```python
from build123d import *

# Parameters (mm, degrees)
F0_W     = 12.7
F0_H     = 44.45
F1_DEPTH = 12.7


with BuildPart() as f1:
    # F0 (on Top) → F1 (new body)
    with BuildSketch(Plane.XY):
        Rectangle(F0_W, F0_H)
        with BuildLine():
            Line((6.35, -22.225), (-6.35, -22.225))
            ThreePointArc((-6.35, -22.225), (-15.875, -31.75), (-25.4, -22.225))
            Line((-25.4, -22.225), (-38.1, -22.225))
            ThreePointArc((-38.1, -22.225), (-15.875, -44.45), (6.35, -22.225))
        make_face()
    extrude(amount=F1_DEPTH)


solid = f1.part
```
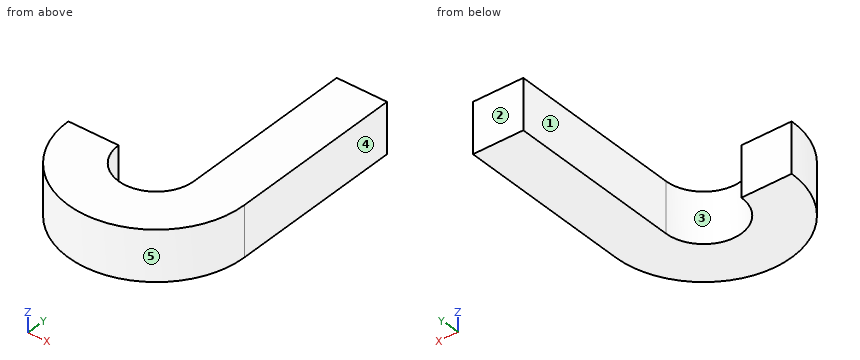
The model under review builds one solid part; all positions refer to its coordinate system, in mm. Face numbers are marked on the shaded views. A direction names the side the tool comes from. Coordinates: 2 decimals unless noted, no trailing zeros. Write each loop counter-clockwise with the first axis right and the second up, starting at its lowest first coordinate (ties: lowest second). Pieces come first, ordered by that corner, then holes.
1) We need section A-A on z = 8. State the section outline as (x, y) points (3 decimals).
2) We need section C-C on x = -2. State the section outline as (y, z) points (3 decimals).
3) The part is to be moulded in two halves that separate along X. For the marked faces 3, 4 and 5, say which applies: pulls with the +X half, pulls with the -X half, needs draft (parallel to the pull), parting line crosses it, or undercut.
4) Machinability: for the marked faces 1 and 2, which of the approach directions +Z, -Z, +X, -X, +Y, -Y give a long, thin tool a straight path to every point of the face, cutting with its end or side? Answer none if there is none.
5) Clearance check with flat-ended pins moving along their axes: pin 1 Ø3 at (x, z) = (-17, 5.5) entering from -Y; pin 2 Ø6 at (y, z) = (-15.5, 4) entering from -X; pin 3 Ø6.5 at (y, z) = (9, 6) entering from -X. State where each tip first meets the part, or that it passes through.
6) We need section B-B on y = -9. State the section outline as (x, z) points.
7) To check wall thickness, follow probe 1 along X at (y, z) = (-5, 10.75); probe 2 along X at (y, z) = (-25, 2); probe 3 along X at (y, z) = (-29, 4.5). State the ranges of each line that lie inside material, in increasing order.
Answer list:
1. outline: (-38.1, -22.225) arc R22.225 ccw to (6.35, -22.225) - (6.35, 22.225) - (-6.35, 22.225) - (-6.35, -22.225) arc R9.525 cw to (-25.4, -22.225) - close
2. outline: (-39.587, 0) - (22.225, 0) - (22.225, 12.7) - (-39.587, 12.7) - close
3. face 3: undercut
3. face 4: pulls with the +X half
3. face 5: parting line crosses it
4. face 1: +Z, -Z, -X, +Y
4. face 2: +Z, -Z, +X, -X, +Y
5. pin 1: stops at y = -44.45
5. pin 2: stops at x = -6.35
5. pin 3: stops at x = -6.35
6. outline: (-6.35, 0) - (6.35, 0) - (6.35, 12.7) - (-6.35, 12.7) - close
7. probe 1: x = -6.35 to 6.35
7. probe 2: x = -37.93 to -24.99, -6.76 to 6.18
7. probe 3: x = -37.04 to -22.57, -9.18 to 5.29
